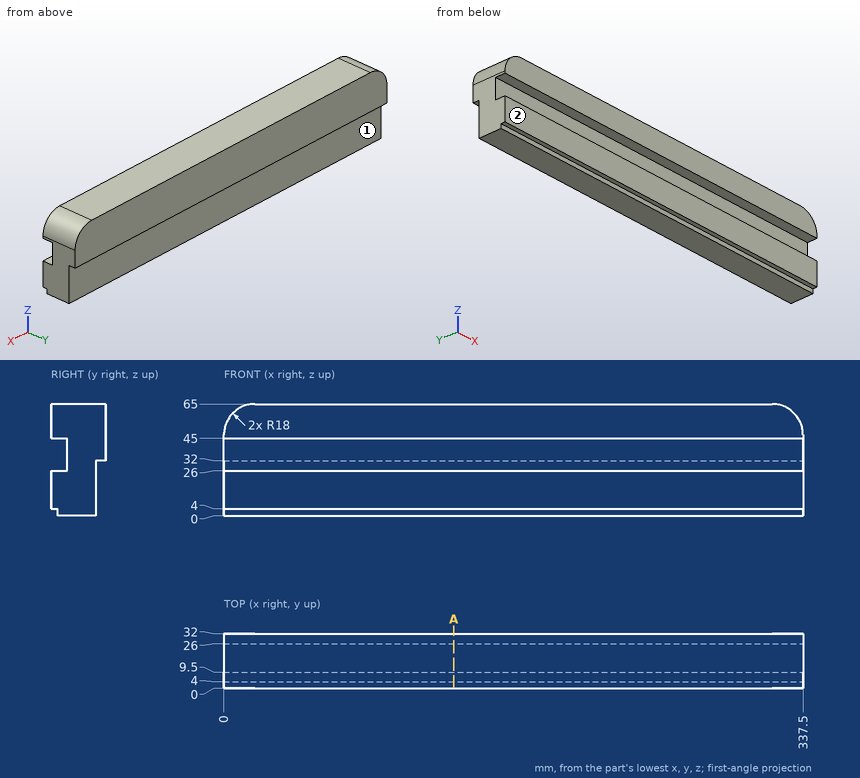
Part print with two shaded views. Sizes in mm from the minimum x, y, z corner. A direction names the side the tool comes from. Round coordinates to 2 decimals unless told otherwise and drop trailing zeros. Loops run counter-clockwise (first coordinate to the right, second up) from the corner with the lowest first, then second, coordinate; pieces in that order, holes last. Notation, with made-up numbers: M -29,43 L 2,43 A13 cw 2,67 Z; hole C -9,-35 d11. An arc over 180 degrees is marked long. Put each result on its own line as item: value. Start each with the question number.
Item 1: Drop flat-ended pins along their axis: P1, Ø4.5, axis at x = 187, y = 1.5, coming from the -Z side; P2, Ø5, axis at x = 86, y = 30, coming from the -Z side; P3, Ø21, axis at x = 177, z = 37.5, coming from the -Y side; P4, Ø4.5, axis at x = 233, z = 1, coming from the -Y side. Give the stop position or say it passes through.
Item 2: Cut at A-A (x = 134). List the corners of the cut face in (y, z).
Item 3: Drill centre lines: line 1 along Z through (x, y) = (265.5, 8); line 2 along Z through (x, y) = (264, 1.5); line 3 along Y through (x, z) = (316.5, 29.5). Where is each one in solid material? Low to high.
Item 4: 3-axis set-ups, long thin cutter, end or side, ignore diameter. For the marked faces 1 and 2: which of +Z, -Z, +X, -X, +Y, -Y reach the whole face in a straight line?
Answer block:
1. P1: z = 4
1. P2: z = 32
1. P3: y = 0
1. P4: y = 4
2. outline: M 0,4 L 4,4 L 4,0 L 26,0 L 26,32 L 32,32 L 32,65 L 0,65 L 0,45 L 9.5,45 L 9.5,26 L 0,26 Z
3. line 1: 0 to 26, 45 to 65
3. line 2: 4 to 26, 45 to 65
3. line 3: 9.5 to 26
4. face 1: -Z, +X, -X, +Y
4. face 2: +Z, -Z, +X, -X, -Y
